Source: CAD feature listing. Evaluate the final solid. Frame: model axes, mm. Face numbers are marked on the shaded views. A direction names the side the tool comes from. Coordinates: 2 decimals unless noted, no trailing zeros. Write each loop counter-clockwise with the first axis right and the second up, starting at its lowest first coordinate (ties: lowest second). Pieces come first, ordered by that corner, then holes. Notation, with made-up numbers: (80, -30) -> (111, -30) arc R19 cw to (111, -7) -> close; hole circle Ø6 at (32, -29). An arc over 180 degrees is marked (long way). Write item = value, one per line.
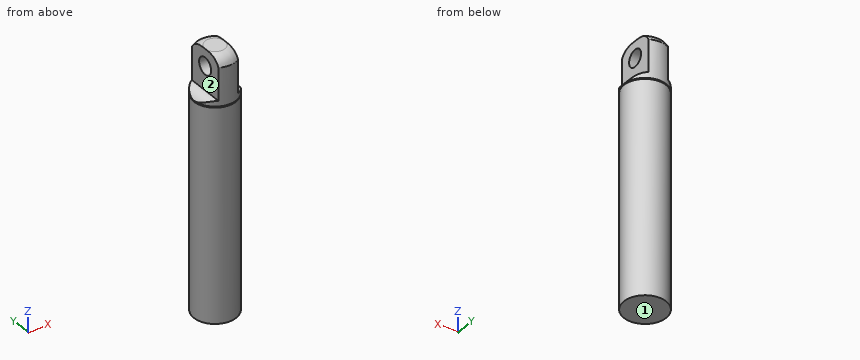
Autodesk Inventor part; units mm, degrees
ref_plane "RodEndPlane" through (0, 0, 50.5) normal (0, 0, 1) x (1, 0, 0)
ref_plane "YZ Plane" through (0, 0, 0) normal (1, 0, 0) x (0, 1, 0)
ref_plane "XZ Plane" through (0, 0, 0) normal (0, 1, 0) x (-1, 0, 0)
sketch "Rod" plane through (0, 0, 0) normal (0, 0, 1) x (1, 0, 0)
  circle A0 centre (0, 0) radius 5
  dimension "d0" = 10
extrude "RodFeature" add sketch "Rod" along normal blind 50.5
ref_plane "RodEndPlane" through (0, 0, 50.5) normal (0, 0, 1) x (1, 0, 0)
sketch "RodEnd" plane through (0, 0, 50.5) normal (0, 0, 1) x (1, 0, 0)
  circle A0 centre (0, 0) radius 5
extrude "RodEndFeature" add sketch "RodEnd" along normal blind 11
sketch "RodEndTip" plane through (0, 0, 0) normal (1, 0, 0) x (0, 1, 0)
  line L0 (5, 0) -> (5, 61.5)
  line L1 (5, 61.5) -> (-5, 61.5)
  line L2 (-5, 0) -> (-5, 61.5)
  arc A0 (5, 59.5) -> (2, 61.5) centre (2.169876, 58.504813) ccw
  line L3 (0, -12.300193) -> (0, 73.801157) construction
  arc A1 (-2, 61.5) -> (-5, 59.5) centre (-2.169876, 58.504813) ccw
  point P0 (0, 0)
  point P1 (-5, 59.5)
  point P2 (-2.339751, 61.5)
  point P3 (2.339751, 61.5)
  dimension "d6" = 3
  dimension "d7" = 2
  dimension "d8" = 3
sketch "RodEndTip outline for RodEndTipFeature" plane through (0, 0, 0) normal (1, 0, 0) x (0, 1, 0)
  arc A0 (-5, 59.5) -> (-2.339751, 61.5) centre (-2.169876, 58.504813) cw
  line L0 (-5, 61.5) -> (-5, 59.5)
  line L1 (-2.339751, 61.5) -> (-5, 61.5)
  arc A1 (2.339751, 61.5) -> (5, 59.5) centre (2.169876, 58.504813) cw
  line L2 (5, 61.5) -> (2.339751, 61.5)
  line L3 (5, 59.5) -> (5, 61.5)
revolve "RodEndTipFeature" cut sketch "RodEndTip outline for RodEndTipFeature" angle 360 about axis through (0, 0, -10) along (0, 0, 1)
sketch "RodEndProfile" plane through (0, 0, 0) normal (0, 1, 0) x (-1, 0, 0)
  line L0 (2.339751, 61.5) -> (-2.339751, 61.5)
  line L1 (-5, 59.5) -> (5, 59.5)
  line L2 (-5, 59.5) -> (5, 59.5)
  line L3 (5, 0) -> (-5, 0)
  line L4 (-2.339751, 61.5) -> (2.339751, 61.5)
  line L5 (2.339751, 61.5) -> (2.339751, 50.5)
  line L6 (2.339751, 50.5) -> (-2.339751, 50.5)
  line L7 (-2.339751, 50.5) -> (-2.339751, 61.5)
  line L8 (-7.423886, 50.5) -> (7.423886, 50.5)
  arc A0 (-2.339751, 61.5) -> (-5, 59.5) centre (-2.169876, 58.504813) ccw
  arc A1 (5, 59.5) -> (2.339751, 61.5) centre (2.169876, 58.504813) ccw
  line L9 (5, 0) -> (5, 59.5)
  line L10 (-5, 0) -> (-5, 59.5)
  arc A2 (5, 50.5) -> (2.339751, 51.83) centre (2.339751, 48.504503) ccw
  line L11 (0, -12.280546) -> (0, 73.683275)
  arc A3 (-2.339751, 51.83) -> (-5, 50.5) centre (-2.339751, 48.504503) ccw
  line L12 (2.339751, 51.83) -> (-2.339751, 51.83) construction
  point P0 (0, 0)
  point P1 (5, 50)
  point P2 (-2.339751, 51.83)
  dimension "d10" = 4.6795
  dimension "d13" = 1.33
extrude "RodEndProfileFeature" cut sketch "RodEndProfile" along normal through all both and the other way through all contours A1 L1 L5 | L1 L9 A2 L5 | L7 L1 A0 | L7 A3 L10 L1
sketch "RodEndEtch" plane through (0, 0, 50.5) normal (0, 0, 1) x (1, 0, 0)
  circle A0 centre (0, 0) radius 5
  circle A1 centre (0, 0) radius 4.75
  dimension "d14" = 0.25
extrude "RodEndEtchFeature" cut sketch "RodEndEtch" against normal blind 0.25
sketch "RodEndHole" plane through (2.339751, -4.418774, 51.83) normal (1, 0, 0) x (0, 0, -1)
  line L0 (64.130968, 4.418774) -> (-21.975807, 4.418774) construction
  line L1 (-3.67, 6.418774) -> (-7.67, 6.418774)
  line L2 (-7.67, 6.418774) -> (-7.67, 2.418774)
  line L3 (-7.67, 2.418774) -> (-3.67, 2.418774)
  line L4 (-3.67, 2.418774) -> (-3.67, 6.418774)
  line L5 (-3.67, 6.418774) -> (-7.67, 2.418774) construction
  line L6 (-7.67, 6.418774) -> (-3.67, 2.418774) construction
  line L7 (-9.67, 4.418774) -> (-9.67, 2.079023)
  point P0 (51.83, 4.418774)
  point P1 (-5.67, 4.418774)
  dimension "d17" = 2
  dimension "d18" = 4
hole "RodEndHoleFeature" at (2.339751, 0, 57.5) direction (-1, 0, 0) diameter 4 end through all
properties part number "1610-50H-2KG-12V-B07-Shaft"
1) Reachability of the marked faces 1 and 2 from +Z, -Z, +X, -X, +Y, -Y: full face, straight path, thin tool, end or side. Return the list, or none.
Answer block:
face_1 = -Z, +X, -X, +Y, -Y
face_2 = +Z, -X, +Y, -Y
2) First-contact query: pin 1 Ø2 at (y, z) = (-3.5, 51.5) entering from +X; pin 2 Ø3 at (x, y) = (1.5, -1) entering from -Z; pin 3 Ø4 at (y, z) = (-4, 30) entering from +X; pin 4 Ø1 at (x, z) = (-3, 30.5) entering from +Y. Flat tips, straight axial feed; report the tip coordinate or a pass-through.
Answer block:
pin_1 = 4.3
pin_2 = 0
pin_3 = 4.58
pin_4 = 4.33
3) Cut plane A-A, the plane z = 57.5. Output: boundary loops of the cut face in (x, y), and give its area (3 significant figures).
Answer block:
outline = (-2.34, -4.42) arc R5 ccw to (2.34, -4.42) -> (2.34, -2) -> (-2.34, -2) -> close; (-2.34, 2) -> (2.34, 2) -> (2.34, 4.42) arc R5 ccw to (-2.34, 4.42) -> close
area = 26.3 mm2
4) Cut plane C-C, the plane z = 13. Output: boundary loops of the cut face in (x, y), and give its area (3 significant figures).
Answer block:
outline = circle Ø10 at (0, 0)
area = 78.5 mm2
5) Material intervals for probe 1 along Z at (x, y) = (1.15, 0); probe 2 along X at (y, z) = (4, 58); probe 3 along X at (y, z) = (-0.25, 23.5), sorted ascending. Write a range as [from, to].
Answer block:
probe_1 = [0, 55.5], [59.5, 61.5]
probe_2 = [-2.34, 2.34]
probe_3 = [-4.99, 4.99]
6) Cut plane D-D, the plane x = -3.5. Output: boundary loops of the cut face in (y, z), and give its area (3 significant figures).
Answer block:
outline = (-3.57, 0) -> (3.57, 0) -> (3.57, 50.25) -> (3.21, 50.25) -> (3.21, 50.5) -> (3.57, 50.5) -> (3.57, 51.62) -> (-3.57, 51.62) -> (-3.57, 50.5) -> (-3.21, 50.5) -> (-3.21, 50.25) -> (-3.57, 50.25) -> close
area = 368 mm2
7) Cut plane B-B, the plane x = 3.75. Output: boundary loops of the cut face in (y, z), and give its area (3 significant figures).
Answer block:
outline = (-3.31, 0) -> (3.31, 0) -> (3.31, 50.25) -> (2.92, 50.25) -> (2.92, 50.5) -> (3.31, 50.5) -> (3.31, 51.52) -> (-3.31, 51.52) -> (-3.31, 50.5) -> (-2.92, 50.5) -> (-2.92, 50.25) -> (-3.31, 50.25) -> close
area = 341 mm2
